from build123d import *

# Parameters (mm, degrees)
BOSS_EXTRUDE1_DEPTH = 4
BOSS_EXTRUDE2_DEPTH = 40
SKETCH3_W           = 25
SKETCH3_H           = 4.000000000000007
BOSS_EXTRUDE3_DEPTH = 20
BOSS_EXTRUDE4_DEPTH = 20
SKETCH5_R           = 2.0000000000000004
SKETCH5_R_2         = 2.0000000000000018
SKETCH5_R_3         = 1.9999999999999967
CUT_EXTRUDE1_DEPTH  = 20
CUT_EXTRUDE3_DEPTH  = 75.00000000000004
SKETCH11_R          = 2.0000000000000027
CUT_EXTRUDE4_DEPTH  = 75.00000000000004
FILLET1_R           = 2
FILLET2_R           = 1
FILLET3_R           = 1
FILLET4_R           = 1
FILLET5_R           = 1
FILLET6_R           = 1
FILLET7_R           = 1
FILLET8_R           = 1
FILLET9_R           = 1
FILLET10_R          = 1
FILLET11_R          = 1
FILLET12_R          = 1
FILLET13_R          = 1
FILLET14_R          = 1
FILLET15_R          = 1
FILLET16_R          = 1
FILLET17_R          = 1
FILLET18_R          = 1
FILLET19_R          = 1
FILLET20_R          = 1
FILLET21_R          = 1


# Some blends are built 0.0001 mm under size
with BuildPart() as part:
    # Sketch1 → Boss-Extrude1 (new body)
    with BuildSketch(Plane(origin=(0, 0, 0), x_dir=(1, 0, 0), z_dir=(0, 1, 0))):
        Polygon((0, 0), (60, 0), (60.00000000000001, -25), (6.94e-15, -25), align=None)
    extrude(amount=BOSS_EXTRUDE1_DEPTH)

    # Sketch2 → Boss-Extrude2 (add)
    with BuildSketch(Plane(origin=(0, 4, 0), x_dir=(1, 0, 0), z_dir=(0, 1, 0))):
        Polygon((0, 0), (4, 0), (4.0000000000000036, -25), (0, -25), align=None)
        Polygon((60, 0), (55.99999999999999, -4.9e-16), (55.99999999999999, -25), (60, -25), align=None)
    extrude(amount=BOSS_EXTRUDE2_DEPTH)

    # Sketch3 → Boss-Extrude3 (add)
    with BuildSketch(Plane(origin=(60, 0, -1.665e-14), x_dir=(-2.8e-16, 0, -1), z_dir=(1, 0, -2.8e-16))):
        with Locations((-12.500000000000018, 42)):
            Rectangle(SKETCH3_W, SKETCH3_H)
    extrude(amount=BOSS_EXTRUDE3_DEPTH)

    # Sketch4 → Boss-Extrude4 (add)
    with BuildSketch(Plane.ZY):
        Polygon((0, 44), (25, 44), (25, 39.99999999999999), (4.9e-16, 39.99999999999999), align=None)
    extrude(amount=BOSS_EXTRUDE4_DEPTH)

    # Sketch5 → Cut-Extrude1 (cut)
    with BuildSketch(Plane(origin=(0, 44, 0), x_dir=(1, 0, 0), z_dir=(0, 1, 0))):
        with Locations(Location((-5.999999999999995, -6.000000000000008, 0), (0, 0, 270))):
            Circle(SKETCH5_R)
        with Locations(Location((-5.9999999999999964, -18.00000000000001, 0), (0, 0, 270))):
            Circle(SKETCH5_R_2)
        with Locations(Location((69.99999999999999, -6.000000000000002, 0), (0, 0, 270))):
            Circle(SKETCH5_R_3)
        with Locations(Location((70, -18.000000000000004, 0), (0, 0, 270))):
            Circle(SKETCH5_R_3)
    extrude(amount=-CUT_EXTRUDE1_DEPTH, mode=Mode.SUBTRACT)

    # Sketch10 → Cut-Extrude3 (cut)
    with BuildSketch(Plane.ZY):
        Polygon((5.148891761902153, 25), (20, 25.000000000000004), (20.000000000000004, 5.0000000000000036), (5.148891761902154, 5.000000000000001), align=None)
    extrude(amount=-CUT_EXTRUDE3_DEPTH, mode=Mode.SUBTRACT)

    # Sketch11 → Cut-Extrude4 (cut)
    with BuildSketch(Plane(origin=(0, 4, 0), x_dir=(1, 0, 0), z_dir=(0, 1, 0))):
        with Locations(Location((14.000000000000005, -12.5, 0), (0, 0, 270))):
            Circle(SKETCH11_R)
        with Locations(Location((45.99999999999999, -12.5, 0), (0, 0, 270))):
            Circle(SKETCH11_R)
    extrude(amount=-CUT_EXTRUDE4_DEPTH, mode=Mode.SUBTRACT)

    # Fillet1
    fillet1_edges = [part.edges().sort_by_distance(p)[0] for p in [
        (-7.999999999999995, 44, 25.000000000000004),
    ]]
    fillet(fillet1_edges, radius=FILLET1_R)

    # Fillet2
    fillet2_edges = [part.edges().sort_by_distance(p)[0] for p in [
        (-19.999999999999996, 44, 11.500000000000002),
        (4.000000000000002, 44, 11.499999999999996),
        (4.0000000000000036, 23, 25),
        (4.0000000000000036, 43.41421356237309, 24.41421356237309),
        (-19.999999999999993, 43.41421356237309, 24.414213562373096),
        (-19.999999999999993, 41, 25.000000000000007),
    ]]
    fillet(fillet2_edges, radius=FILLET2_R)

    # Fillet3
    fillet3_edges = [part.edges().sort_by_distance(p)[0] for p in [
        (68, 44, 25),
    ]]
    fillet(fillet3_edges, radius=FILLET3_R)

    # Fillet4
    fillet4_edges = [part.edges().sort_by_distance(p)[0] for p in [
        (55.99999999999999, 23.5, 25),
        (55.99999999999999, 43.707106781186546, 24.707106781186546),
        (55.99999999999999, 44, 12),
    ]]
    fillet(fillet4_edges, radius=FILLET4_R)

    # Fillet5
    fillet5_edges = [part.edges().sort_by_distance(p)[0] for p in [
        (30, 4, 25),
    ]]
    fillet(fillet5_edges, radius=FILLET5_R)

    # Fillet6
    fillet6_edges = [part.edges().sort_by_distance(p)[0] for p in [
        (3.49e-15, 5.000000000000002, 12.574445880951078),
    ]]
    fillet(fillet6_edges, radius=FILLET6_R)

    # Fillet7
    fillet7_edges = [part.edges().sort_by_distance(p)[0] for p in [
        (1.32e-15, 14.5, 5.148891761902153),
    ]]
    fillet(fillet7_edges, radius=FILLET7_R)

    # Fillet8
    fillet8_edges = [part.edges().sort_by_distance(p)[0] for p in [
        (3.33e-15, 25, 12.074445880951076),
    ]]
    fillet(fillet8_edges, radius=FILLET8_R)

    # Fillet9
    fillet9_edges = [part.edges().sort_by_distance(p)[0] for p in [
        (3.78e-15, 19.999999999999996, 25),
    ]]
    fillet(fillet9_edges, radius=FILLET9_R)

    # Fillet10
    fillet10_edges = [part.edges().sort_by_distance(p)[0] for p in [
        (55.99999999999999, 5.000000000000003, 12.574445880951062),
    ]]
    fillet(fillet10_edges, radius=FILLET10_R - 0.0001)  # a hair under: the kernel refuses the full size

    # Fillet11
    fillet11_edges = [part.edges().sort_by_distance(p)[0] for p in [
        (55.99999999999999, 14.500050000000002, 5.148891761902138),
    ]]
    fillet(fillet11_edges, radius=FILLET11_R)

    # Fillet12
    fillet12_edges = [part.edges().sort_by_distance(p)[0] for p in [
        (55.99999999999999, 25, 12.074445880951062),
    ]]
    fillet(fillet12_edges, radius=FILLET12_R)

    # Fillet13
    fillet13_edges = [part.edges().sort_by_distance(p)[0] for p in [
        (55.99999999999999, 15.000050000000003, 19.999999999999986),
    ]]
    fillet(fillet13_edges, radius=FILLET13_R)

    # Fillet14
    fillet14_edges = [part.edges().sort_by_distance(p)[0] for p in [
        (30.500000000000007, 0, 25),
        (0.2928932188134594, -1.1e-16, 24.707106781186546),
        (3.33e-15, 0, 12),
    ]]
    fillet(fillet14_edges, radius=FILLET14_R)

    # Fillet15
    fillet15_edges = [part.edges().sort_by_distance(p)[0] for p in [
        (29.999999999999996, 4, 0),
    ]]
    fillet(fillet15_edges, radius=FILLET15_R)

    # Fillet16
    fillet16_edges = [part.edges().sort_by_distance(p)[0] for p in [
        (0, 20.499999999999996, 0),
        (0.2928932188134523, 0.2928932188134522, 2e-16),
        (56.29289321881345, 43.707106781186546, 0),
        (30.5, 0, 0),
        (60, 19.999999999999996, 0),
        (80, 42, -5.55e-15),
        (70, 39.99999999999999, -2.78e-15),
        (68.5, 44, -2.66e-15),
        (55.99999999999999, 23, -1.1e-16),
    ]]
    fillet(fillet16_edges, radius=FILLET16_R)

    # Fillet17
    fillet17_edges = [part.edges().sort_by_distance(p)[0] for p in [
        (3.7071067811865475, 43.707106781186546, -1e-16),
        (-20, 41.5, 5.86e-15),
        (-19.707106781186546, 43.707106781186546, 2e-16),
        (4, 23, -1.1e-16),
        (-8, 44, 2.78e-15),
    ]]
    fillet(fillet17_edges, radius=FILLET17_R)

    # Fillet18
    fillet18_edges = [part.edges().sort_by_distance(p)[0] for p in [
        (-8.999999999999996, 39.99999999999999, 25),
        (-19.70710678118654, 39.99999999999999, 24.707106781186546),
        (-19.999999999999996, 39.99999999999999, 12.499999999999998),
        (-19.707106781186546, 39.99999999999999, 0.29289321881345254),
        (-9, 39.99999999999999, 2.99e-15),
    ]]
    fillet(fillet18_edges, radius=FILLET18_R)

    # Fillet19
    # the kernel refuses this fillet: 1 mm, written as the material it takes off along each edge
    with BuildSketch(Plane(origin=(79, 43, 1), x_dir=(1, 0, -2.8e-16), z_dir=(0, 1, 0))) as fillet19_piece_1_section:
        Polygon((0, 0), (FILLET19_R * 1.02, 0), (FILLET19_R * 1.02, FILLET19_R * 1.02), (2.8e-16, FILLET19_R * 1.02), align=None)
    fillet19_piece_1 = extrude(amount=FILLET19_R * 1.02, mode=Mode.PRIVATE)
    fillet19_piece_1 = fillet19_piece_1 - Plane(origin=(79, 43, 1), x_dir=(-0.7071067811865475, 0, 0.7071067811865477), z_dir=(0, 1, 0)) * Sphere(FILLET19_R, mode=Mode.PRIVATE)
    add(fillet19_piece_1, mode=Mode.SUBTRACT)
    with BuildSketch(Plane(origin=(79, 40.99999999999999, 1.0000000000000002), x_dir=(0, -1, 0), z_dir=(1, 0, -2.8e-16))) as fillet19_piece_2_section:
        Polygon((0, 0), (FILLET19_R * 1.02, 0), (FILLET19_R * 1.02, FILLET19_R * 1.02), (0, FILLET19_R * 1.02), align=None)
    fillet19_piece_2 = extrude(amount=FILLET19_R * 1.02, mode=Mode.PRIVATE)
    fillet19_piece_2 = fillet19_piece_2 - Plane(origin=(79, 40.99999999999999, 1.0000000000000002), x_dir=(0, 0.7071067811865475, 0.7071067811865475), z_dir=(1, 0, -2.8e-16)) * Sphere(FILLET19_R, mode=Mode.PRIVATE)
    add(fillet19_piece_2, mode=Mode.SUBTRACT)
    with BuildSketch(Plane(origin=(80, 37.49999999999999, 25), x_dir=(-1, 0, 0), z_dir=(0, 1, 0))) as fillet19_piece_3:
        with BuildLine():
            CenterArc((FILLET19_R, -FILLET19_R), FILLET19_R, 90, 90)
            Line((0, -FILLET19_R), (0, 0))
            Line((0, 0), (FILLET19_R, 0))
        make_face()
    extrude(amount=5.500000000000007, mode=Mode.SUBTRACT)
    with BuildSketch(Plane(origin=(80, 43, 23.999999999999996), x_dir=(0, 0, 1), z_dir=(0, -1, 0))) as fillet19_piece_4:
        with BuildLine():
            CenterArc((1 - FILLET19_R, FILLET19_R), FILLET19_R, 270, 90)
            Line((1 - FILLET19_R, 0), (1, 0))
            Line((1, 0), (1, FILLET19_R))
        make_face()
    revolve(axis=Axis((80, 43, 23.999999999999996), (-1, 0, 1.5e-16)), revolution_arc=90, mode=Mode.SUBTRACT)
    with BuildSketch(Plane(origin=(80, 44, 23.999999999999996), x_dir=(-1, 0, 2.8e-16), z_dir=(-2.8e-16, 0, -1))) as fillet19_piece_5:
        with BuildLine():
            CenterArc((FILLET19_R, -FILLET19_R), FILLET19_R, 90, 90)
            Line((0, -FILLET19_R), (0, 0))
            Line((0, 0), (FILLET19_R, 0))
        make_face()
    extrude(amount=22.999999999999996, mode=Mode.SUBTRACT)
    with BuildSketch(Plane(origin=(80, 39.99999999999999, 0.9999999999999998), x_dir=(0, 1, 0), z_dir=(2.8e-16, 0, 1))) as fillet19_piece_6:
        with BuildLine():
            CenterArc((FILLET19_R, FILLET19_R), FILLET19_R, 180, 90)
            Line((0, FILLET19_R), (0, 0))
            Line((0, 0), (FILLET19_R, 0))
        make_face()
    extrude(amount=26.499999999999996, mode=Mode.SUBTRACT)

    # Fillet20
    fillet20_edges = [part.edges().sort_by_distance(p)[0] for p in [
        (60, 15, 5.148891761902136),
        (60, 25.000000000000004, 12.57444588095106),
        (60.00000000000001, 15.000000000000004, 19.999999999999986),
        (60, 5.000000000000003, 12.574445880951062),
    ]]
    fillet(fillet20_edges, radius=FILLET20_R)

    # Fillet21
    fillet21_edges = [part.edges().sort_by_distance(p)[0] for p in [
        (4.000000000000001, 15, 5.148891761902152),
        (4.000000000000002, 25.000000000000004, 12.574445880951075),
        (4.000000000000003, 15.000000000000004, 20),
        (4.000000000000002, 5.000000000000003, 12.574445880951076),
    ]]
    fillet(fillet21_edges, radius=FILLET21_R - 0.0001)  # a hair under: the kernel refuses the full size


solid = part.part
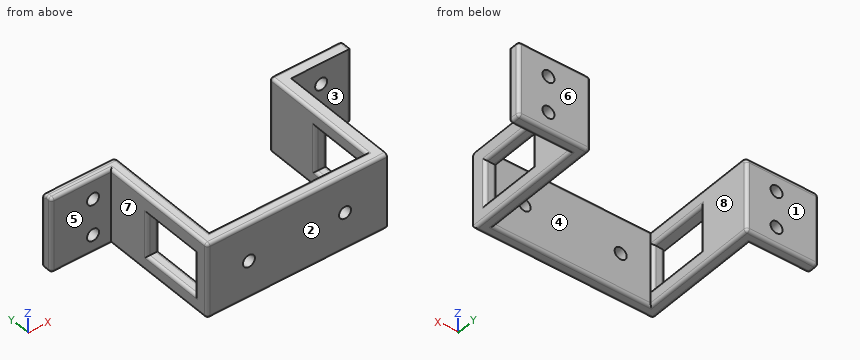
Here's how the part is built. I have some questions about the finished solid (model axes, mm). Face numbers are marked on the shaded views. A direction names the side the tool comes from. Give positions to 0.01 mm unless a question says otherwise; leave off trailing zeros. Order: outer loops, then holes, each group sorted by start corner. A loop starts at its lowest first (then second) coordinate and runs counter-clockwise, first axis right, second up. Notation, with made-up numbers: (-14, -38) -> (22, -38) arc R19 cw to (22, -29) -> close; hole circle Ø6 at (16, 16.5). An arc over 180 degrees is marked (long way). Use a Markdown table: item, result. Add a question column.
Item 1: I need wall thicknesses on line 1 (X direction, y = 1.15, z = 12.5); line 2 (X direction, y = 40.9, z = 6); line 3 (X direction, y = 29, z = 23.25). Which ranges of each line are inside material? Lowest first, please.
Item 2: For the marked faces 1, 2, 3, 4 and 5, which set-ups out of +Z, -Z, +X, -X, +Y, -Y let a thin tool reach every point of the face, with its end or its side?
Item 3: Will these pins go through, and if not, where does the flat tip stop? pin 1 (4 mm diameter, centred on x = 44, z = 9, fed in from +Y); pin 2 (2 mm diameter, centred on x = 65, z = 3.5, fed in from -Y); pin 3 (10 mm diameter, centred on y = 31.5, z = 11.5, fed in from +X).
Item 4: Imagine slicing it at D-D on x = -6. Please give me the cut outline in (y, z), plus the area to 3 significant figures.
Item 5: Imagine slicing it at C-C on y = 6. Give the number of separate pieces and of enclosed holes in the cut face, plus the area to 3 significant figures.
Item 6: Imagine slicing it at B-B on x = 14. Please give me the cut outline in (y, z), plus the area to 3 significant figures.
Item 7: Imagine slicing it at A-A on y = 30.5. Please give me the cut outline in (x, z).
Item 8: If we mould it in two halves opening along X, with no side actions, what happens to the marked faces 6, 7 and 8? For each: pulls with the +X half, pulls with the -X half, needs draft (parallel to the pull), parting line crosses it, or undercut.
Data:
| question | item | result |
|---|---|---|
| 1 | line 1 | x = 0 to 12, 16 to 44, 48 to 60 |
| 1 | line 2 | x = -19.99 to -8, -4 to 4, 56 to 68, 72 to 79.99 |
| 1 | line 3 | x = 0 to 4, 56 to 60 |
| 2 | face 1 | +Z, -Z, +X, -X, +Y |
| 2 | face 2 | +Z, -Z, +X, -X, -Y |
| 2 | face 3 | +Z, -Z, +X, -Y |
| 2 | face 4 | +Z, -Z, +Y |
| 2 | face 5 | +Z, -Z, -X, -Y |
| 3 | pin 1 | stops at y = 4 |
| 3 | pin 2 | stops at y = 40 |
| 3 | pin 3 | stops at x = 60 |
| 4 | outline | (40, 1) arc R1 ccw to (41, 0) -> (43, 0) arc R1 ccw to (44, 1) -> (44, 4) -> (40, 4) -> close; (40, 8) -> (44, 8) -> (44, 16) -> (40, 16) -> close; (40, 20) -> (44, 20) -> (44, 23) arc R2 ccw to (42, 25) -> (41, 25) arc R1 ccw to (40, 24) -> close |
| 4 | area | 66.5 mm² |
| 5 | separate pieces | 4 |
| 5 | enclosed holes | 0 |
| 5 | area | 78.2 mm² |
| 6 | outline | (0, 1) arc R1 ccw to (1, 0) -> (3, 0) arc R1 ccw to (4, 1) -> (4, 10.5) -> (0, 10.5) -> close; (0, 14.5) -> (4, 14.5) -> (4, 24) arc R1 ccw to (3, 25) -> (1, 25) arc R1 ccw to (0, 24) -> close |
| 6 | area | 83.1 mm² |
| 7 | outline | (0, 1) arc R1 ccw to (1, 0) -> (3, 0) arc R1 ccw to (4, 1) -> (4, 24) arc R1 ccw to (3, 25) -> (1, 25) arc R1 ccw to (0, 24) -> close; (56, 1) arc R1 ccw to (57, 0) -> (59, 0) arc R1 ccw to (60, 1) -> (60, 25) -> (57, 25) arc R1 ccw to (56, 24) -> close |
| 8 | face 6 | needs draft |
| 8 | face 7 | pulls with the -X half |
| 8 | face 8 | undercut |
